For this review, take the finished solid that the model builds, in its own axes (mm). A direction names the side the tool comes from. Coordinates: 2 decimals unless noted, no trailing zeros. Write each loop counter-clockwise with the first axis right and the second up, starting at its lowest first coordinate (ties: lowest second). Pieces come first, ordered by that corner, then holes.
1) To check wall thickness, follow line 1 along Z through (x, y) = (161.5, -51); line 2 along Y through (x, z) = (-49.5, 31); line 3 along Y through (x, z) = (150, 82.2). State the ranges of each line that lie inside material, in increasing order.
2) We need section B-B on x = 79. Write out the cut boundary in (y, z).
3) For faces 4 (the face through (-154, 87, 82)), 5 (the face through (107.04, -105.8, 41.45)), 6 (the face through (-117.98, 53.56, 1.48)), list the 3-axis set-ups (+Z, -Z, +X, -X, +Y, -Y) from which the entire face can be reached by the end or side of a thin tool; tool diameter is ignored.
4) Insertion check: P1, Ø1.5, axis at y = -152.5, z = 49, coming from the +X side; P2, Ø8, axis at x = 11.5, z = 71.5, coming from the +Y side; P3, Ø5.5, axis at x = 10.5, z = 89, coming from the -Y side. Each pin has a flat end and moves straight along its axis. Give the tip position at first contact, or say it passes through.
5) Mouldability with a two-part tool opening along Z and no side actions: class faces 1 (the face through (170, 10, 91)), 2 (the face through (-49.68, 112.45, 1.48)), 3 (the face through (103, 119, 3)) as pulls with the +Z half, pulls with the -Z half, needs draft (parallel to the pull), parting line crosses it, or undercut.
6) We need section C-C on y = -33. Write out the cut boundary in (x, z).
7) We need section D-D on y = -90. Give the number of separate pieces and of enclosed holes in the cut face, then the cut area to 3 significant figures.
from build123d import *

# Parameters (mm, degrees)
SKETCH_R           = 200
SKETCH_R_2         = 100
SKETCH_R_3         = 5
PAD_DEPTH          = 3
SKETCH001_W        = 3
SKETCH001_H        = 126
PAD001_DEPTH       = 84
SKETCH002_R        = 200
SKETCH002_R_2      = 127
SKETCH002_R_3      = 5
PAD002_DEPTH       = 3
POLARPATTERN_COUNT = 8
SKETCH003_W        = 20
SKETCH003_H        = 20
PAD003_DEPTH       = 10


with BuildPart() as part:
    # Sketch → Pad (new body)
    with BuildSketch(Plane.XY):
        Circle(SKETCH_R)
        Circle(SKETCH_R_2, mode=Mode.SUBTRACT)
        with Locations((-117.332701, 48.600796)):
            Circle(SKETCH_R_3, mode=Mode.SUBTRACT)
        with Locations((-48.600796, 117.332701)):
            Circle(SKETCH_R_3, mode=Mode.SUBTRACT)
        with Locations((48.600796, 117.332701)):
            Circle(SKETCH_R_3, mode=Mode.SUBTRACT)
        with Locations((117.332701, 48.600796)):
            Circle(SKETCH_R_3, mode=Mode.SUBTRACT)
        with Locations((117.332701, -48.600796)):
            Circle(SKETCH_R_3, mode=Mode.SUBTRACT)
        with Locations((48.600796, -117.332701)):
            Circle(SKETCH_R_3, mode=Mode.SUBTRACT)
        with Locations((-48.600796, -117.332701)):
            Circle(SKETCH_R_3, mode=Mode.SUBTRACT)
        with Locations((-117.332701, -48.600796)):
            Circle(SKETCH_R_3, mode=Mode.SUBTRACT)
    extrude(amount=PAD_DEPTH)

    # Sketch001 → Pad001 (join)
    with BuildSketch(Plane.XY):
        with Locations((-152, 0)):
            Rectangle(SKETCH001_W, SKETCH001_H)
    pad001 = extrude(amount=PAD001_DEPTH)

    # Sketch002 (on DatumPlane) → Pad002 (join)
    with BuildSketch(Plane.XY.offset(81)):
        Circle(SKETCH002_R)
        Circle(SKETCH002_R_2, mode=Mode.SUBTRACT)
        with Locations((-150, 90)):
            Circle(SKETCH002_R_3, mode=Mode.SUBTRACT)
        with Locations((-150, -90)):
            Circle(SKETCH002_R_3, mode=Mode.SUBTRACT)
        with Locations((150, 90)):
            Circle(SKETCH002_R_3, mode=Mode.SUBTRACT)
        with Locations((150, -90)):
            Circle(SKETCH002_R_3, mode=Mode.SUBTRACT)
    extrude(amount=PAD002_DEPTH)

    # PolarPattern: Pad001 ×8 about axis
    polarpattern_axis = Axis((0, 0, 0), (0, 0, 1))
    for i in range(1, POLARPATTERN_COUNT):
        add(pad001.rotate(polarpattern_axis, i * 360 / POLARPATTERN_COUNT))

    # Sketch003 (on DatumPlane) → Pad003 (join)
    with BuildSketch(Plane.XY.offset(81)):
        with Locations((170, 10)):
            Rectangle(SKETCH003_W, SKETCH003_H)
        with Locations((-10, 170)):
            Rectangle(SKETCH003_W, SKETCH003_H)
        with Locations((-170, -10)):
            Rectangle(SKETCH003_W, SKETCH003_H)
        with Locations((10, -170)):
            Rectangle(SKETCH003_W, SKETCH003_H)
    extrude(amount=PAD003_DEPTH)


solid = part.part
Result:
1. line 1: z = 0 to 3, 81 to 84
1. line 2: y = -153.5 to -150.5, 150.5 to 153.5
1. line 3: y = -132.29 to -95, -85 to 85, 95 to 132.29
2. outline: (-183.74, 0) - (-61.31, 0) - (-61.31, 3) - (-133.84, 3) - (-133.84, 81) - (-99.44, 81) - (-99.44, 84) - (-183.74, 84) - (-183.74, 81) - (-138.08, 81) - (-138.08, 3) - (-183.74, 3) - close; (61.31, 0) - (183.74, 0) - (183.74, 3) - (138.08, 3) - (138.08, 81) - (183.74, 81) - (183.74, 84) - (99.44, 84) - (99.44, 81) - (133.84, 81) - (133.84, 3) - (61.31, 3) - close
3. face 4: +Z
3. face 5: none
3. face 6: -Z
4. P1: stops at x = 65.33
4. P2: stops at y = 153.5
4. P3: stops at y = -180
5. face 1: pulls with the +Z half
5. face 2: needs draft
5. face 3: undercut
6. outline: (-197.26, 0) - (-94.4, 0) - (-94.4, 3) - (-150.5, 3) - (-150.5, 81) - (-122.64, 81) - (-122.64, 84) - (-197.26, 84) - (-197.26, 81) - (-153.5, 81) - (-153.5, 3) - (-197.26, 3) - close; (94.4, 0) - (197.26, 0) - (197.26, 3) - (153.5, 3) - (153.5, 81) - (197.26, 81) - (197.26, 84) - (122.64, 84) - (122.64, 81) - (150.5, 81) - (150.5, 3) - (94.4, 3) - close
7. separate pieces: 4
7. enclosed holes: 0
7. area: 1,950 mm2
